Part print with two shaded views. Sizes in mm from the minimum x, y, z corner. Round coordinates to 2 decimals unless told otherwise and drop trailing zeros. Order: outer loops, then holes, each group sorted by start corner. A loop starts at its lowest first (then second) coordinate and runs counter-clockwise, first axis right, second up. Notation, with made-up numbers: (-27, 82) - (19, 82) arc R8 cw to (19, 88) - close; hole circle Ø11 at (19.5, 9). An arc over 180 degrees is marked (long way). Use one line per item in the form item = value.
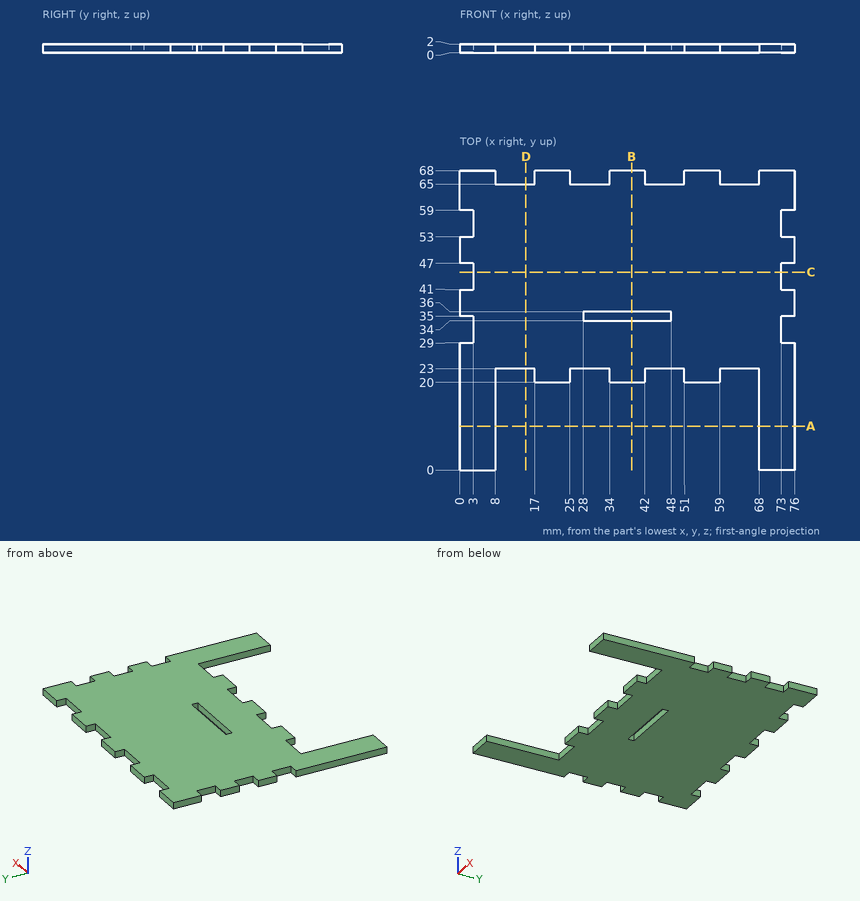
(1) Slice it at D-D on x = 15. Give the cut face in (y, z).
Report:
outline = (23, 0) - (65, 0) - (65, 2) - (23, 2) - close
(2) Probe probe 1 along X at (y, z) = (18, 0.75); probe 2 along Y at (x, z) = (32, 0.6); probe 3 along X at (y, z) = (46, 1.05). List the from-to ranges inside material, lowest first. Write a range as [from, to].
Report:
probe_1 = [0, 8], [68, 76]
probe_2 = [23, 34], [36, 65]
probe_3 = [3, 73]
(3) Slice it at B-B on x = 39. Give the cut face in (y, z), then the cut area to 3 significant figures.
Report:
outline = (20, 0) - (34, 0) - (34, 2) - (20, 2) - close; (36, 0) - (68, 0) - (68, 2) - (36, 2) - close
area = 92.0 mm2
(4) Pin check, flat tip, straight feed: pin 1 (1 mm diameter, centred on x = 46.5, z = 1, fed in from +Y). Stop position of the tip, or through.
Report:
pin_1 = 65
(5) Slice it at C-C on y = 45. Give the cut face in (x, z), then the cut area to 3 significant figures.
Report:
outline = (3, 0) - (73, 0) - (73, 2) - (3, 2) - close
area = 140 mm2
(6) Slice it at A-A on y = 10. Give the cut face in (x, z), then the cut area to 3 significant figures.
Report:
outline = (0, 0) - (8, 0) - (8, 2) - (0, 2) - close; (68, 0) - (76, 0) - (76, 2) - (68, 2) - close
area = 32.0 mm2
